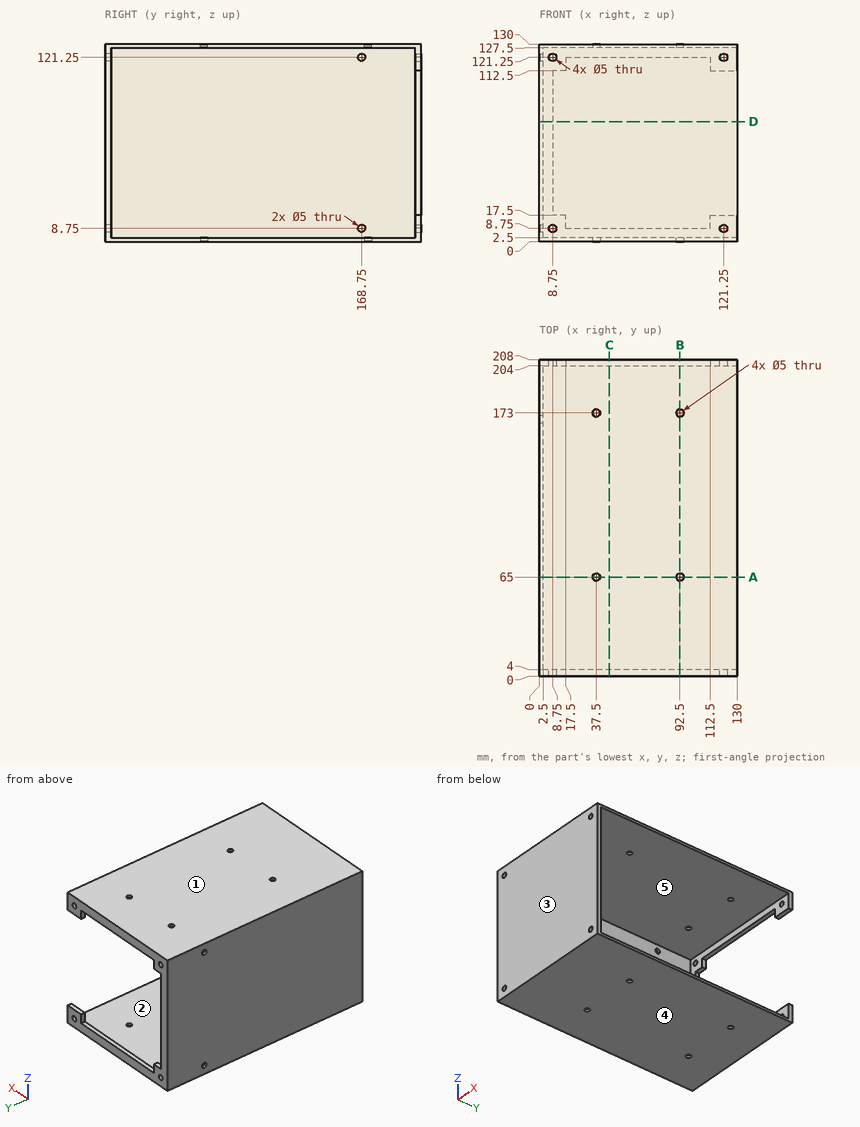
Job drawing, mm, ordinate dimensions from the low corner. One solid piece. A direction names the side the tool comes from. Coordinates: 2 decimals unless noted, no trailing zeros. Loops run counter-clockwise (first coordinate to the right, second up) from the corner with the lowest first, then second, coordinate; pieces in that order, holes last. Notation, with made-up numbers: (-15, 25.5) - (12, 25.5) arc R30 cw to (12, 54.5) - close; hole circle Ø10 at (86.5, -14). An arc over 180 degrees is marked (long way). Answer as a JSON object with one key per item and string values. Group by question number.
(1) Tool access for the marked faces 1 and 2: list every direction of +Z, -Z, +X, -X, +Y, -Y with a clear straight run to the whole face (end or side of a thin tool).
(2) Probe line 1 along Z through (x, y) = (121.25, 0.85); line 2 along Y through (x, z) = (92.5, 128.1); line 3 along X through (y, z) = (65, 128). List the from-to ranges inside material, lowest first.
(3) Two-plate mould, pull along Y, no slides. Class the marked faces 3, 4 and 5: released by +Y, released by -Y, zero draft, split by the parting line, or undercut.
(4) Cut at B-B (x = 92.5). Give the cut face in (y, z).
(5) Cut at D-D (z = 79). Give the cut face in (x, y).
(6) Cut at C-C (x = 46). Give the cut face in (y, z).
(7) Flat gauge pins, fed straight in: pin 1 (5 mm diameter, centred on y = 183, z = 42.5, fed in from +X); pin 2 (12 mm diameter, centred on x = 96.5, z = 17, fed in from +Y). Where does each tip first touch, or does it go through?
(8) Cut at A-A (y = 65). Give the cut face in (x, z).
Geometry says:
{
 "1": {"face 1": "+Z, +X, -X, +Y, -Y", "face 2": "+X"},
 "2": {"line 1": "z = 0 to 6.25, 11.25 to 118.75, 123.75 to 130", "line 2": "y = 0 to 62.5, 67.5 to 170.5, 175.5 to 208", "line 3": "x = 0 to 35, 40 to 90, 95 to 130"},
 "3": {"face 3": "released by -Y", "face 4": "zero draft", "face 5": "undercut"},
 "4": {"outline": "(0, 0) - (62.5, 0) - (62.5, 2.5) - (4, 2.5) - (4, 127.5) - (62.5, 127.5) - (62.5, 130) - (0, 130) - close; (67.5, 0) - (170.5, 0) - (170.5, 2.5) - (67.5, 2.5) - close; (67.5, 127.5) - (170.5, 127.5) - (170.5, 130) - (67.5, 130) - close; (175.5, 0) - (208, 0) - (208, 8.75) - (204, 8.75) - (204, 2.5) - (175.5, 2.5) - close; (175.5, 127.5) - (204, 127.5) - (204, 121.25) - (208, 121.25) - (208, 130) - (175.5, 130) - close"},
 "5": {"outline": "(0, 0) - (130, 0) - (130, 4) - (2.5, 4) - (2.5, 204) - (8.75, 204) - (8.75, 208) - (0, 208) - close"},
 "6": {"outline": "(0, 0) - (208, 0) - (208, 8.75) - (204, 8.75) - (204, 2.5) - (4, 2.5) - (4, 127.5) - (204, 127.5) - (204, 121.25) - (208, 121.25) - (208, 130) - (0, 130) - close"},
 "7": {"pin 1": "stops at x = 2.5", "pin 2": "stops at y = 4"},
 "8": {"outline": "(0, 0) - (35, 0) - (35, 2.5) - (2.5, 2.5) - (2.5, 127.5) - (35, 127.5) - (35, 130) - (0, 130) - close; (40, 0) - (90, 0) - (90, 2.5) - (40, 2.5) - close; (40, 127.5) - (90, 127.5) - (90, 130) - (40, 130) - close; (95, 0) - (130, 0) - (130, 2.5) - (95, 2.5) - close; (95, 127.5) - (130, 127.5) - (130, 130) - (95, 130) - close"}
}
